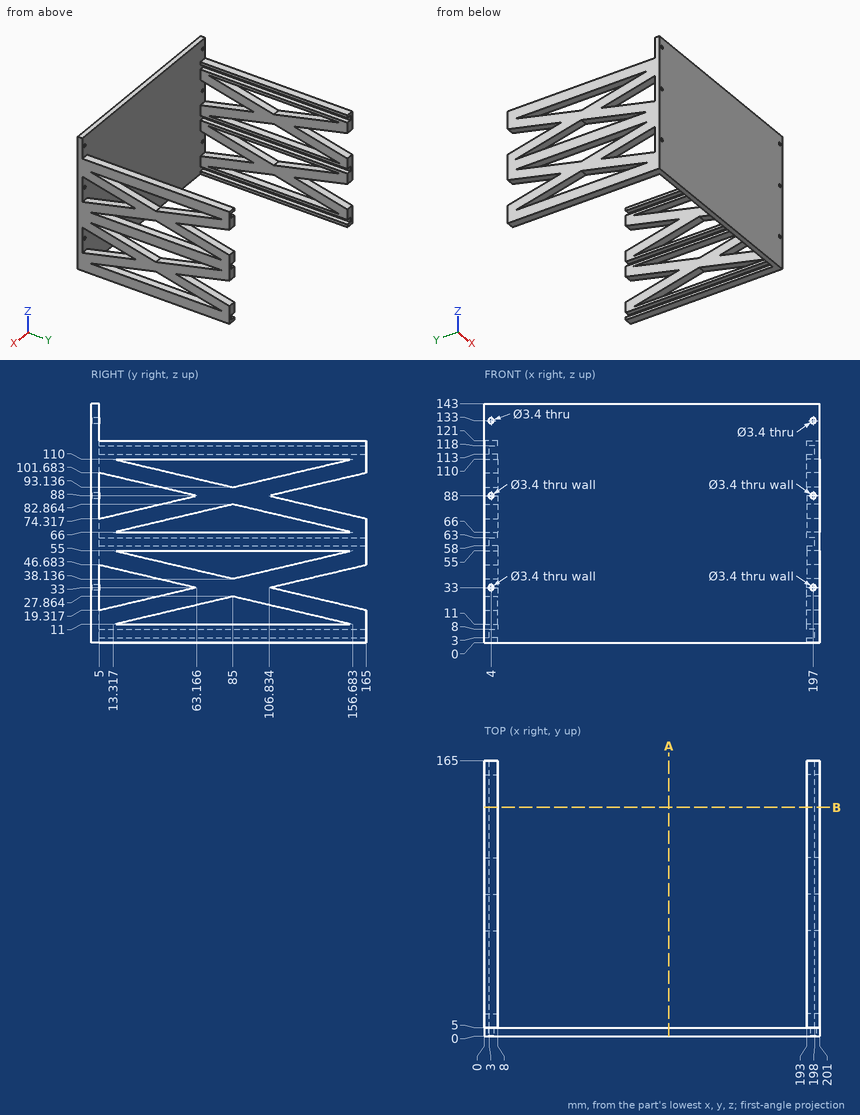
Source: three-view drawing plus pictorial views. Frame: mm from the lowest corner of the part. Give positions to 0.01 mm unless a question says otherwise; leave off trailing zeros. Write each loop counter-clockwise with the first axis right and the second up, starting at its lowest first coordinate (ties: lowest second). Pieces come first, ordered by that corner, then holes.
(1) Cut plane A-A, the plane x = 110.5. Return loops of the section in (y, z), then the cut area to 3 significant figures.
(2) Ray query, line 1 (X direction, y = 4, z = 33); line 2 (Z direction, x = 197, y = 2.45); line 3 (X direction, y = 114, z = 7). Return the intervals inside material, ascending.
(3) First-contact query: P1, Ø2.5, axis at x = 3, y = 61.5, coming from the +Z side; P2, Ø2, axis at x = 34.5, z = 109.5, coming from the +Y side. Flat tips, straight axial feed; report the tip coordinate or a pass-through.
(4) Cut plane B-B, the plane y = 137. Give the number of separate pieces and of enclosed holes in the cut face.
Values follow:
1. outline: (0, 0) - (5, 0) - (5, 143) - (0, 143) - close
1. area: 715 mm2
2. line 1: x = 0 to 2.3, 5.7 to 195.3, 198.7 to 201
2. line 2: z = 0 to 31.3, 34.7 to 86.3, 89.7 to 131.3, 134.7 to 143
2. line 3: x = 0 to 3, 198 to 201
3. P1: stops at z = 121
3. P2: stops at y = 5
4. separate pieces: 14
4. enclosed holes: 0
